from build123d import *

# Parameters (mm, degrees)
SKETCH_1_R          = 6.1
EXTRUDE_1_DEPTH     = 10.2
EXTRUDE_START       = 5
EXTRUDE_2_DEPTH     = 3.9
CUT_EXTRUDE_START   = 2.1
CUT_EXTRUDE_1_DEPTH = 5
CUT_EXTRUDE_2_DEPTH = 12.83342723
SKETCH_4_R          = 4.5
EXTRUDE_3_DEPTH     = 4.3
SKETCH_5_R          = 3
CUT_EXTRUDE_3_DEPTH = 2.1
SKETCH_6_R          = 4
SKETCH_6_R_2        = 3.5
EXTRUDE_4_DEPTH     = 1.5
SKETCH_6_2_R        = 3.5
EXTRUDE_5_DEPTH     = 5.4


with BuildPart() as part:
    # Sketch 1 → Extrude 1 (new body)
    with BuildSketch(Plane.XY):
        Circle(SKETCH_1_R)
    extrude(amount=EXTRUDE_1_DEPTH)

    # Sketch 1_5 → Extrude 2 (add)
    with BuildSketch(Plane.XY.offset(EXTRUDE_START)):
        with BuildLine():
            Line((-5.25, -3.106042498), (-5.25, -5.25))
            Line((-5.25, -5.25), (-3.106042498, -5.25))
            ThreePointArc((-3.106042498, -5.25), (-4.313351365, -4.313351365), (-5.25, -3.106042498))
        make_face()
        with BuildLine():
            ThreePointArc((5.25, -3.106042498), (4.313351365, -4.313351365), (3.106042498, -5.25))
            Line((3.106042498, -5.25), (5.25, -5.25))
            Line((5.25, -5.25), (5.25, -3.106042498))
        make_face()
        with BuildLine():
            Line((-5.25, 5.25), (-5.25, 3.106042498))
            ThreePointArc((-5.25, 3.106042498), (-4.313351365, 4.313351365), (-3.106042498, 5.25))
            Line((-3.106042498, 5.25), (-5.25, 5.25))
        make_face()
        with BuildLine():
            ThreePointArc((3.106042498, 5.25), (4.313351365, 4.313351365), (5.25, 3.106042498))
            Line((5.25, 3.106042498), (5.25, 5.25))
            Line((5.25, 5.25), (3.106042498, 5.25))
        make_face()
    extrude(amount=EXTRUDE_2_DEPTH)

    # Sketch 1_6 → Cut-Extrude 1 (cut)
    with BuildSketch(Plane.XY.offset(CUT_EXTRUDE_START)):
        with BuildLine():
            Line((5.25, 3.106042498), (5.25, -3.106042498))
            ThreePointArc((5.25, -3.106042498), (5.883663825, -1.610124219), (6.1, 0))
            ThreePointArc((6.1, 0), (5.883663825, 1.610124219), (5.25, 3.106042498))
        make_face()
        with BuildLine():
            ThreePointArc((-5.25, 3.106042498), (-6.1, 0), (-5.25, -3.106042498))
            Line((-5.25, -3.106042498), (-5.25, 3.106042498))
        make_face()
    extrude(amount=CUT_EXTRUDE_1_DEPTH, mode=Mode.SUBTRACT)

    # Sketch 3 → Cut-Extrude 2 (cut, through all)
    with BuildSketch(Plane.XY.offset(2.1)):
        Polygon((-10.9126982, 1.5), (-10.9126982, -1.5), (-5.9126982, -1.5), (-5.25, -1.5), (-5.25, 1.5), (-5.9126982, 1.5), align=None)
        with BuildLine():
            Line((5.9126982, 1.5), (5.25, 1.5))
            Line((5.25, 1.5), (5.25, -1.5))
            Line((5.25, -1.5), (5.9126982, -1.5))
            ThreePointArc((5.9126982, -1.5), (6.1, 0), (5.9126982, 1.5))
        make_face()
    extrude(amount=-CUT_EXTRUDE_2_DEPTH, mode=Mode.SUBTRACT)

    # Sketch 4 → Extrude 3 (add)
    with BuildSketch(Plane(origin=(0, 0, 0), x_dir=(-1, 0, 0), z_dir=(0, 0, -1))):
        with Locations(Location((0, 0, 0), (0, 0, 180))):
            Circle(SKETCH_4_R)
    extrude(amount=EXTRUDE_3_DEPTH)

    # Sketch 5 → Cut-Extrude 3 (cut)
    with BuildSketch(Plane(origin=(0, 0, -4.3), x_dir=(-1, 0, 0), z_dir=(0, 0, -1))):
        Circle(SKETCH_5_R)
    extrude(amount=-CUT_EXTRUDE_3_DEPTH, mode=Mode.SUBTRACT)

    # Sketch 6 → Extrude 4 (add)
    with BuildSketch(Plane.XY.offset(10.2)):
        Circle(SKETCH_6_R)
        Circle(SKETCH_6_R_2, mode=Mode.SUBTRACT)
    extrude(amount=EXTRUDE_4_DEPTH)

    # Sketch 6_2 → Extrude 5 (add)
    with BuildSketch(Plane.XY.offset(10.2)):
        with Locations(Location((0, 0, 0), (0, 0, 180))):
            Circle(SKETCH_6_2_R)
    extrude(amount=EXTRUDE_5_DEPTH)


solid = part.part
Read the model definition and answer for the solid it produces. Units are mm, in the model's axes. A direction names the side the tool comes from. Round coordinates to 2 decimals unless told otherwise and drop trailing zeros. Order: outer loops, then holes, each group sorted by start corner. A loop starts at its lowest first (then second) coordinate and runs counter-clockwise, first axis right, second up.
1) Flat-ended cylindrical pins translate along their axes: pin 1 (3 mm diameter, centred on y = 4.5, z = 11.5, fed in from -X); pin 2 (1.7 mm diameter, centred on x = -4.5, y = 4, fed in from +Z); pin 3 (1.1 mm diameter, centred on x = -4.5, z = 6.5, fed in from -Y); pin 4 (4.5 mm diameter, centred on y = -0.5, z = 5, fed in from -X). Find the tip coordinate at first contact, or state that the pin passes through.
2) Straight lines are drawn through the part: L1, parallel to Y at x = 0, z = -3.1; L2, parallel to Z at x = 4.25, y = -4.75; L3, parallel to Z at x = -2.25, y = 1. For each, find the intervals that lie inside material, in ascending order.
3) The part is cut by section B-B on x = 0. Write down the section's boundary in (y, z), plus the area to 3 significant figures.
4) For faces 4 (the face through (0, 5, 0)), 5 (the face through (4, -1.3, 10.2)), 6 (the face through (-5, -5, 8.9)), determine the directions among +Z, -Z, +X, -X, +Y, -Y from which every point of the face is accessible in a straight line to the end or side of a thin tool.
5) The part is cut by section A-A on y = 0. Write down the section's boundary in (x, z).
6) The part is cut by section D-D on z = 12.5. Write down the section's boundary in (x, y), plus the area to 3 significant figures.
7) The mould has two halves that part along Z. Classify faces 1 (the face through (-3.32, -3.04, -2.12)), 2 (the face through (-5.6, 0, 7.1)), 3 (the face through (-5, 5, 5)): released by +Z, released by -Z, zero draft, split by the parting line, or undercut.
8) The part is cut by section C-C on z = -3. Write down the section's boundary in (x, y), plus the area to 3 significant figures.
Resolved:
1. pin 1: stops at x = -4.81
1. pin 2: stops at z = 10.2
1. pin 3: stops at y = -5.25
1. pin 4: stops at x = -6.1
2. L1: y = -4.5 to -3, 3 to 4.5
2. L2: z = 5 to 8.9
2. L3: z = -2.2 to 15.6
3. outline: (-6.1, 0) - (-4.5, 0) - (-4.5, -4.3) - (-3, -4.3) - (-3, -2.2) - (3, -2.2) - (3, -4.3) - (4.5, -4.3) - (4.5, 0) - (6.1, 0) - (6.1, 10.2) - (4, 10.2) - (4, 11.7) - (3.5, 11.7) - (3.5, 15.6) - (-3.5, 15.6) - (-3.5, 11.7) - (-4, 11.7) - (-4, 10.2) - (-6.1, 10.2) - close
3. area: 190 mm2
4. face 4: -Z
4. face 5: +Z
4. face 6: +Z, -X, -Y
5. outline: (-6.1, 7.1) - (-5.25, 7.1) - (-5.25, 0) - (-4.5, 0) - (-4.5, -4.3) - (-3, -4.3) - (-3, -2.2) - (3, -2.2) - (3, -4.3) - (4.5, -4.3) - (4.5, 0) - (5.25, 0) - (5.25, 7.1) - (6.1, 7.1) - (6.1, 10.2) - (4, 10.2) - (4, 11.7) - (3.5, 11.7) - (3.5, 15.6) - (-3.5, 15.6) - (-3.5, 11.7) - (-4, 11.7) - (-4, 10.2) - (-6.1, 10.2) - close
6. outline: circle Ø7 at (0, 0)
6. area: 38.5 mm2
7. face 1: zero draft
7. face 2: undercut
7. face 3: released by -Z
8. outline: circle Ø9 at (0, 0); hole circle Ø6 at (0, 0)
8. area: 35.3 mm2
